Verification items for the finished model (mm, model axes). A direction names the side the tool comes from. Round coordinates to 2 decimals unless told otherwise and drop trailing zeros. Write each loop counter-clockwise with the first axis right and the second up, starting at its lowest first coordinate (ties: lowest second). Pieces come first, ordered by that corner, then holes. Notation, with made-up numbers: M -8,67.5 L 27,67.5 A8 cw 27,76.5 Z; hole C -12,43 d4. An arc over 180 degrees is marked long. Answer in a Markdown table with one row per item. Add a question column.
1. Sectioned sample at C-C on x = 40. Record the cut outline in (y, z).
2. Go/stop test with flat-tipped pins: pin 1 Ø4 at (x, y) = (-30.5, -1) entering from -Z; pin 2 Ø1 at (y, z) = (8.5, 1) entering from +X; pin 3 Ø0.6 at (x, z) = (11.5, 1.5) entering from -Y; pin 4 Ø4 at (x, y) = (30, 0) entering from -Z. Record where each tip stops, or that it passes through.
3. Material ranges on probe 1 along X at (y, z) = (2, 1); probe 2 along Y at (x, z) = (-30, -3.75); probe 3 along Y at (x, z) = (3.5, 0.75), recorded low to high.
4. Sectioned sample at B-B on y = -33. Record the cut outline in (x, z).
5. Sectioned sample at D-D on y = 0. Record the cut outline in (x, z).
6. Sectioned sample at A-A on x = -30. Record the cut outline in (y, z), plus the area to 3 significant figures.
7. Set-up check for faces 1 (the cylindrical face through (32.5, 0.1, -3.5)), 2 (the cylindrical face through (-72.15, -46.99, -2.46)), 3 (the flat face through (-1, 1, 0)): record each of +Z, -Z, +X, -X, +Y, -Y from which the full face is reachable in a straight line by a thin tool's end or side.
```python
from build123d import *

# Parameters (mm, degrees)
BOSS_EXTRUDE1_DEPTH = 5
SKETCH2_W           = 130
SKETCH2_H           = 80
SKETCH2_W_2         = 126
SKETCH2_H_2         = 76
BOSS_EXTRUDE2_DEPTH = 2
FILLET1_R           = 1
SKETCH3_R           = 2.5
CUT_EXTRUDE1_DEPTH  = 3


with BuildPart() as part:
    # Sketch1 → Boss-Extrude1 (new body)
    with BuildSketch(Plane.XY):
        with BuildLine():
            Line((65, 50), (-65, 50))
            ThreePointArc((-65, 50), (-72.071067812, 47.071067812), (-75, 40))
            Line((-75, 40), (-75, -40))
            ThreePointArc((-75, -40), (-72.071067812, -47.071067812), (-65, -50))
            Line((-65, -50), (65, -50))
            ThreePointArc((65, -50), (72.071067812, -47.071067812), (75, -40))
            Line((75, -40), (75, 40))
            ThreePointArc((75, 40), (72.071067812, 47.071067812), (65, 50))
        make_face()
    extrude(amount=-BOSS_EXTRUDE1_DEPTH)

    # Sketch2 → Boss-Extrude2 (add)
    with BuildSketch(Plane.XY):
        Rectangle(SKETCH2_W, SKETCH2_H)
        Rectangle(SKETCH2_W_2, SKETCH2_H_2, mode=Mode.SUBTRACT)
    extrude(amount=BOSS_EXTRUDE2_DEPTH)

    # Fillet1
    fillet1_edges = [part.edges().sort_by_distance(p)[0] for p in [
        (0, -40, 0),
        (65, 0, 2),
        (-65, 0, 2),
        (0, 40, 2),
    ]]
    fillet(fillet1_edges, radius=FILLET1_R - 0.0001)  # a hair under: the kernel refuses the full size

    # Sketch3 → Cut-Extrude1 (cut)
    with BuildSketch(Plane(origin=(0, 0, -5), x_dir=(-1, 0, 0), z_dir=(0, 0, -1))):
        with Locations((-30, 0)):
            Circle(SKETCH3_R)
        with Locations((30, 0)):
            Circle(SKETCH3_R)
    extrude(amount=-CUT_EXTRUDE1_DEPTH, mode=Mode.SUBTRACT)


solid = part.part
```
Geometry check:
| question | item | result |
|---|---|---|
| 1 | outline | M -50,-5 L 50,-5 L 50,0 L 40,0 L 40,1 A1 ccw 39,2 L 38,2 L 38,0 L -38,0 L -38,2 L -40,2 L -40,1 A1 cw -41,0 L -50,0 Z |
| 2 | pin 1 | stops at z = -5 |
| 2 | pin 2 | stops at x = 65 |
| 2 | pin 3 | stops at y = -40 |
| 2 | pin 4 | stops at z = -2 |
| 3 | probe 1 | x = -65 to -63, 63 to 65 |
| 3 | probe 2 | y = -50 to -2.5, 2.5 to 50 |
| 3 | probe 3 | y = -40.03 to -38, 38 to 40 |
| 4 | outline | M -75,-5 L 75,-5 L 75,0 L 65,0 L 65,1 A1 ccw 64,2 L 63,2 L 63,0 L -63,0 L -63,2 L -64,2 A1 ccw -65,1 L -65,0 L -75,0 Z |
| 5 | outline | M -75,-5 L -32.5,-5 L -32.5,-2 L -27.5,-2 L -27.5,-5 L 27.5,-5 L 27.5,-2 L 32.5,-2 L 32.5,-5 L 75,-5 L 75,0 L 65,0 L 65,1 A1 ccw 64,2 L 63,2 L 63,0 L -63,0 L -63,2 L -64,2 A1 ccw -65,1 L -65,0 L -75,0 Z |
| 6 | outline | M -50,-5 L -2.5,-5 L -2.5,-2 L 2.5,-2 L 2.5,-5 L 50,-5 L 50,0 L 40,0 L 40,1 A1 ccw 39,2 L 38,2 L 38,0 L -38,0 L -38,2 L -40,2 L -40,1 A1 cw -41,0 L -50,0 Z |
| 6 | area | 493 mm2 |
| 7 | face 1 | -Z |
| 7 | face 2 | +Z, -Z, -X, -Y |
| 7 | face 3 | +Z |
